Part print with two shaded views. Sizes in mm from the minimum x, y, z corner. Give positions to 0.01 mm unless a question says otherwise; leave off trailing zeros. Loops run counter-clockwise (first coordinate to the right, second up) from the corner with the lowest first, then second, coordinate; pieces in that order, holes last. Notation, with made-up numbers: M -36,29 L -19,29 A24 ccw -19,60 Z; hole C -22.5,-20.75 d9. An arc over 180 degrees is marked long. Answer in a Markdown table with one row per item.
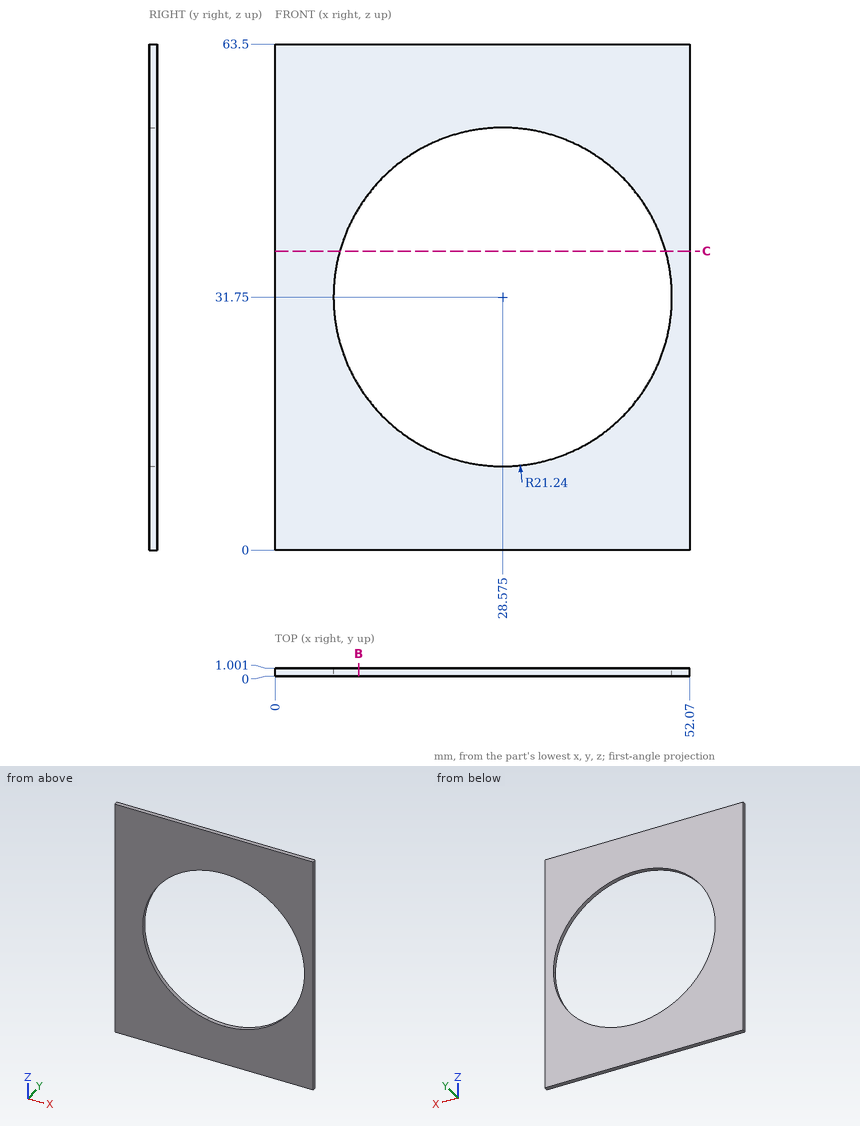
Q1. Probe probe 1 along Z at (x, y) = (47, 0.9) (1 decimal); probe 2 along Z at (x, y) = (10, 0.45); probe 3 along X at (y, z) = (0.8, 16.5). List the from-to ranges inside material, lowest first.
Reported:
| item | result |
|---|---|
| probe 1 | 0 to 21.2, 42.3 to 63.5 |
| probe 2 | 0 to 21.45, 42.05 to 63.5 |
| probe 3 | 0 to 13.79, 43.36 to 52.07 |
Q2. Saw through at B-B (x = 10.5). Give the cut face in (y, z) (1 decimal).
Reported:
| item | result |
|---|---|
| outline | M 0,0 L 1,0 L 1,20.6 L 0,20.6 Z; M 0,42.9 L 1,42.9 L 1,63.5 L 0,63.5 Z |
Q3. Saw through at C-C (z = 37.5). Give the cut face in (x, y).
Reported:
| item | result |
|---|---|
| outline | M 0,0 L 8.13,0 L 8.13,1 L 0,1 Z; M 49.02,0 L 52.07,0 L 52.07,1 L 49.02,1 Z |
